```python
from build123d import *

# Parameters (mm, degrees)
PAD005_DEPTH    = 9
THICKNESS001_T  = -1
POCKET003_DEPTH = 1
POCKET004_DEPTH = 1


with BuildPart() as part:
    # Sketch008 → Pad005 (new body)
    with BuildSketch(Plane.XY):
        Polygon((20.318948, 34.5), (27.318948, 34.5), (27.318948, 54.5), (47.318948, 54.5), (47.318948, 34.5), (54.318948, 34.5), (54.318948, -34.5), (20.318948, -34.5), align=None)
    extrude(amount=PAD005_DEPTH)

    # Thickness001
    thickness001_openings = [part.faces().sort_by_distance(p)[0] for p in [
        (37.318948, 6.482156, 9),
    ]]
    offset(amount=THICKNESS001_T, openings=thickness001_openings)

    # Sketch009 (on Face3 of Thickness001) → Pocket003 (cut)
    with BuildSketch(Plane(origin=(0, 54.5, 0), x_dir=(-1, 0, 0), z_dir=(0, 1, 0))):
        with BuildLine():
            ThreePointArc((-40.318948, 9), (-43.318948, 12), (-46.318948, 9))
            Line((-46.318948, 9), (-46.318948, 5))
            ThreePointArc((-46.318948, 5), (-43.318948, 2), (-40.318948, 5))
            Line((-40.318948, 9), (-40.318948, 5))
        make_face()
    extrude(amount=-POCKET003_DEPTH, mode=Mode.SUBTRACT)

    # Sketch010 (on Face10 of Pocket003) → Pocket004 (cut)
    with BuildSketch(Plane.YZ.offset(54.318948)):
        with BuildLine():
            ThreePointArc((23.5, 1.5), (31, 9), (23.5, 16.5))
            Line((23.5, 16.5), (-23.5, 16.5))
            ThreePointArc((-23.5, 16.5), (-31, 9), (-23.5, 1.5))
            Line((23.5, 1.5), (-23.5, 1.5))
        make_face()
    extrude(amount=-POCKET004_DEPTH, mode=Mode.SUBTRACT)


solid = part.part
```
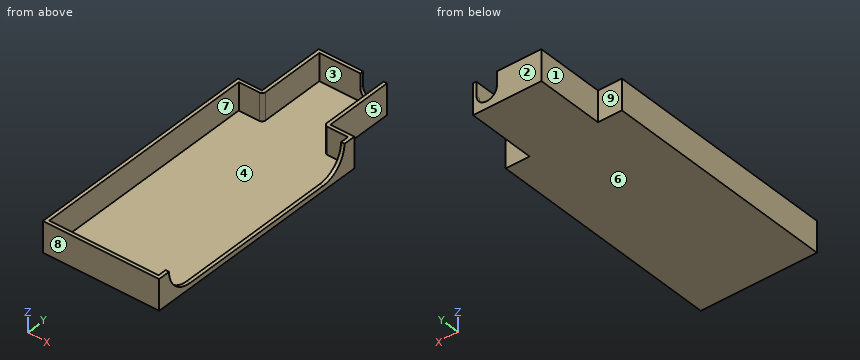
The model under review builds one solid part; all positions refer to its coordinate system, in mm. Face numbers are marked on the shaded views. A direction names the side the tool comes from. Round coordinates to 2 decimals unless told otherwise and drop trailing zeros. Loops run counter-clockwise (first coordinate to the right, second up) from the corner with the lowest first, then second, coordinate; pieces in that order, holes last. Notation, with made-up numbers: (-39, 42) - (17, 42) arc R15 ccw to (17, 46) - close; hole circle Ø6 at (-18, -33). An arc over 180 degrees is marked (long way). Use a Markdown table: item, result. Add a question column.
Q1. Add section A-A (z = 7). State the section outline as (x, y) points.
Q2. For probe 1 along Y at (x, z) = (31.5, 1.25); probe 2 along X at (y, z) = (-29.5, 3.25); probe 3 along Y at (x, z) = (53, 6.25), list the stretches that pass through material, from the lowest coordinate up.
Q3. Add section C-C (x = 48.5). State the section outline as (y, z) points, plus the area to 3 significant figures.
Q4. Machinability: for the marked faces 5, 6, 7, 8 and 9, which of the approach directions +Z, -Z, +X, -X, +Y, -Y give a long, thin tool a straight path to every point of the face, cutting with its end or side? Answer none if there is none.
Q5. The part is to be moulded in two halves that separate along X. For the marked faces 1, 2, 3 and 4, say which applies: pulls with the +X half, pulls with the -X half, needs draft (parallel to the pull), parting line crosses it, or undercut.
Q6. Add section B-B (y = -3.5). State the section outline as (x, z) points, plus the area to 3 significant figures.
Q7. Insertion check: pin 1 Ø16 at (x, y) = (34, 26.5) entering from +Z; pin 2 Ø1.1 at (x, y) = (53.5, 6.5) entering from +Z; pin 3 Ø4 at (y, z) = (-16, 4) entering from +X. Each pin has a flat end and moves straight along its axis. Give the tip position at first contact, or say it passes through.
Worked answers:
| question | item | result |
|---|---|---|
| 1 | outline | (20.32, -34.5) - (54.32, -34.5) - (54.32, -30.73) - (53.32, -30.73) - (53.32, -33.5) - (21.32, -33.5) - (21.32, 33.5) - (27.32, 33.5) arc R1 ccw to (28.32, 34.5) - (28.32, 53.5) - (40.32, 53.5) - (40.32, 54.5) - (27.32, 54.5) - (27.32, 34.5) - (20.32, 34.5) - close; (46.32, 34.5) arc R1 ccw to (47.32, 33.5) - (53.32, 33.5) - (53.32, 30.73) - (54.32, 30.73) - (54.32, 34.5) - (47.32, 34.5) - (47.32, 54.5) - (46.32, 54.5) - close |
| 2 | probe 1 | -34.5 to -33.5, 53.5 to 54.5 |
| 2 | probe 2 | 20.32 to 21.32, 53.32 to 54.32 |
| 2 | probe 3 | -34.5 to -33.5, 33.5 to 34.5 |
| 3 | outline | (-34.5, 0) - (34.5, 0) - (34.5, 9) - (33.5, 9) - (33.5, 1) - (-33.5, 1) - (-33.5, 9) - (-34.5, 9) - close |
| 3 | area | 85.0 mm² |
| 4 | face 5 | +Z, -Z, +X, +Y |
| 4 | face 6 | -Z, +X, -X, +Y, -Y |
| 4 | face 7 | +Z |
| 4 | face 8 | +Z, -Z, +X, -X, -Y |
| 4 | face 9 | +Z, -Z, -X, +Y |
| 5 | face 1 | pulls with the -X half |
| 5 | face 2 | needs draft |
| 5 | face 3 | undercut |
| 5 | face 4 | undercut |
| 6 | outline | (20.32, 0) - (54.32, 0) - (54.32, 1.5) - (53.32, 1.5) - (53.32, 1) - (21.32, 1) - (21.32, 9) - (20.32, 9) - close |
| 6 | area | 42.5 mm² |
| 7 | pin 1 | z = 1 |
| 7 | pin 2 | z = 1.5 |
| 7 | pin 3 | x = 21.32 |
